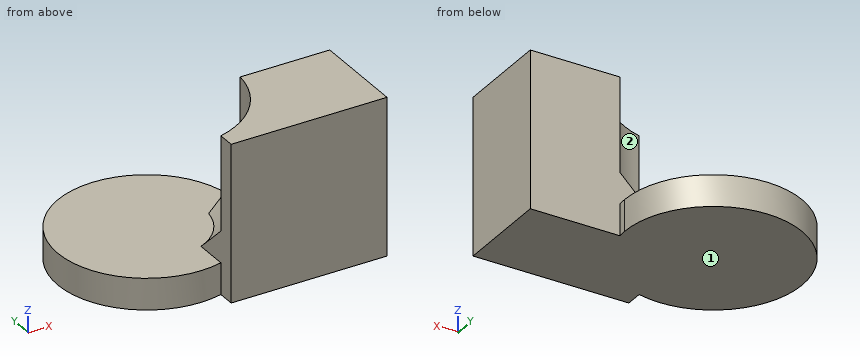
```python
from build123d import *

# Parameters (mm, degrees)
F1_DEPTH    = 25.4
F2_DEPTH    = 5.08
F3_T4_ANGLE = 174.1930400009


# Not quite as in the source:
# - a fillet or chamfer that OpenCascade refuses, or shapes differently, is made with other operations: its cross-section is extruded or revolved along the edge and cut away or added


with BuildPart() as f1:
    # F0 (on Top) → F1 (new body)
    with BuildSketch(Plane.XY):
        with BuildLine():
            Line((-28.7617053837, 23.086078465), (-43.2633440317, 23.086078465))
            ThreePointArc((-43.2633440317, 23.086078465), (-46.6420182582, 15.0906140017), (-54.0029779077, 10.4907048123))
            Line((-54.0029779077, 10.4907048123), (-54.0029779077, 7.7324733138))
            Line((-54.0029779077, 7.7324733138), (-28.7617053837, 7.7324733138))
            Line((-28.7617053837, 7.7324733138), (-28.7617053837, 23.086078465))
        make_face()
    extrude(amount=F1_DEPTH)

    # F0 (on Top) → F2 (join)
    with BuildSketch(Plane.XY):
        with BuildLine():
            Line((-54.0029779077, 10.4907048123), (-54.0029779077, 23.086078465))
            Line((-54.0029779077, 23.086078465), (-43.2633440317, 23.086078465))
            ThreePointArc((-43.2633440317, 23.086078465), (-43.2161007803, 23.7580355867), (-43.2003415292, 24.4314670563))
            ThreePointArc((-43.2003415292, 24.4314670563), (-68.9767505511, 33.249655712), (-54.0029779077, 10.4907048123))
        make_face()
        with BuildLine():
            Line((-43.2633440317, 23.086078465), (-54.0029779077, 23.086078465))
            Line((-54.0029779077, 23.086078465), (-54.0029779077, 10.4907048123))
            ThreePointArc((-54.0029779077, 10.4907048123), (-46.6420182582, 15.0906140017), (-43.2633440317, 23.086078465))
        make_face()
    extrude(amount=F2_DEPTH)

    # F3: chamfer of 5.08 on 1 edges, made by hand


with BuildPart() as f3_tool2:
    # F3_s3 → F3_t4 (revolve)
    with BuildSketch(Plane(origin=(-48.0088326829, 36.9045281739, 0), x_dir=(0, 0, 1), z_dir=(-0.7928262046, 0.6094477905, 0))):
        Polygon((10.16, -30.128971911), (5.08, -25.048971911), (5.08, -30.128971911), align=None)
    revolve(axis=Axis((-57.5969107449, 24.4314670563, 5.08), (0, 0, 1)), revolution_arc=F3_T4_ANGLE)

    split(bisect_by=Plane.XZ.offset(-23.086078465), keep=Keep.TOP)

    split(bisect_by=Plane.YZ.offset(-54.0029779077), keep=Keep.TOP)


with BuildPart() as f1_1:
    add(f1.part)

    # F3_t1: union F3_tool2
    add(f3_tool2.part)


solid = f1_1.part
```
Verification items for the finished model (mm, model axes). Face numbers are marked on the shaded views. A direction names the side the tool comes from. Give positions to 0.01 mm unless a question says otherwise; leave off trailing zeros. Write each loop counter-clockwise with the first axis right and the second up, starting at its lowest first coordinate (ties: lowest second). Pieces come first, ordered by that corner, then holes. Notation, with made-up numbers: M 34,48 L 86,48 A25 cw 86,80 Z; hole C -24,-34.75 d9. An arc over 180 degrees is marked long. One line per question, with ' | ' between items.
1) Set-up check for the marked faces 1 and 2: record each of +Z, -Z, +X, -X, +Y, -Y from which the full face is reachable in a straight line by a thin tool's end or side.
Result:
face 1: -Z, +X, -X, +Y, -Y | face 2: +Z, -X, +Y
2) Thickness scan on line 1 along Z through (x, y) = (-54, 31); line 2 along Y through (x, z) = (-31, 19.5); line 3 along X through (y, z) = (16, 8.25). Record the ranges inside material, lowest first. Write a range as [from, to].
Result:
line 1: z = [0, 5.08] | line 2: y = [7.73, 23.09] | line 3: x = [-48.39, -28.76]
3) Section check C-C on y = 34. Enter the section's corners in (x, z).
Result:
outline: M -68.35,0 L -46.84,0 L -46.84,5.08 L -68.35,5.08 Z
4) Section check B-B on x = -39.5. Enter the section's corners in (y, z).
Result:
outline: M 7.73,0 L 23.09,0 L 23.09,25.4 L 7.73,25.4 Z
5) Section check A-A on z = 10.75. Enter the section's corners in (x, y).
Result:
outline: M -54,7.73 L -28.76,7.73 L -28.76,23.09 L -43.26,23.09 A14.4 cw -54,10.49 Z
6) Gauge pin test, flat ends, axial feed: pin 1 Ø5 at (x, z) = (-59, 13) entering from -Y; pin 2 Ø9 at (y, z) = (13, 7) entering from -X; pin 3 Ø10 at (x, y) = (-66, 17.5) entering from +Z; pin 4 Ø10 at (x, z) = (-37, 14) entering from +Y. Record the tip position at first contact, or that the pin passes through.
Result:
pin 1: passes through | pin 2: stops at x = -69.97 | pin 3: stops at z = 5.08 | pin 4: stops at y = 23.09
